Check sheet for the modelled part. Datum: model origin and axes. Units: mm. Face numbers are marked on the shaded views. A direction names the side the tool comes from. Coordinates: 2 decimals unless noted, no trailing zeros. Order: outer loops, then holes, each group sorted by start corner. A loop starts at its lowest first (then second) coordinate and runs counter-clockwise, first axis right, second up.
1. Draft check along Z on the marked faces 1, 2, 3 and 4. Enter one of: released by +Z, released by -Z, zero draft, split by the parting line, or undercut.
2. Cross-section at C-C (y = -49). Enter the section's corners in (x, z).
3. Gauge pin test, flat ends, axial feed: pin 1 Ø6 at (y, z) = (-22, 7) entering from +X; pin 2 Ø4 at (x, y) = (-5.5, -38) entering from -Z; pin 3 Ø1.5 at (y, z) = (-6.5, -3) entering from +X. Record the tip position at first contact, or that the pin passes through.
4. Set-up check for the marked faces 5 and 6: record each of +Z, -Z, +X, -X, +Y, -Y from which the full face is reachable in a straight line by a thin tool's end or side.
5. Cross-section at A-A (z = 0). Enter the section's corners in (x, y).
6. Cross-section at D-D (x = 6.75). Enter the section's corners in (y, z).
7. Cross-section at B-B (x = 0). Enter the section's corners in (y, z), then the cut area to 3 significant figures.
8. Thickness scan on line 1 (Z direction, x = 0, y = -0.1); line 2 (Z direction, x = 0, y = -17); line 3 (Y direction, x = 9.75, z = -3.5). Record the ranges inside material, lowest first.
```python
from build123d import *

# Parameters (mm, degrees)
F0_R     = 12
F1_DEPTH = 57.5
F2_R     = 7.5
F3_DEPTH = 2
F4_R     = 7.5
F5_DEPTH = 54
F6_R     = 4.25
F7_DEPTH = 8


with BuildPart() as f1:
    # F0 (on Front) → F1 (new body)
    with BuildSketch(Plane.XZ):
        Circle(F0_R)
    extrude(amount=F1_DEPTH)

    # F2 (on face) → F3 (join)
    with BuildSketch(Plane(origin=(0, 0, 0), x_dir=(-1, 0, 0), z_dir=(0, 1, 0))):
        Circle(F2_R)
    extrude(amount=F3_DEPTH)

    # F4 (on face) → F5 (cut)
    with BuildSketch(Plane.XZ.offset(57.5)):
        Circle(F4_R)
    extrude(amount=-F5_DEPTH, mode=Mode.SUBTRACT)

    # F6 (on face) → F7 (cut)
    with BuildSketch(Plane(origin=(0, 2, 0), x_dir=(-1, 0, 0), z_dir=(0, 1, 0))):
        Circle(F6_R)
    extrude(amount=-F7_DEPTH, mode=Mode.SUBTRACT)


solid = f1.part
```
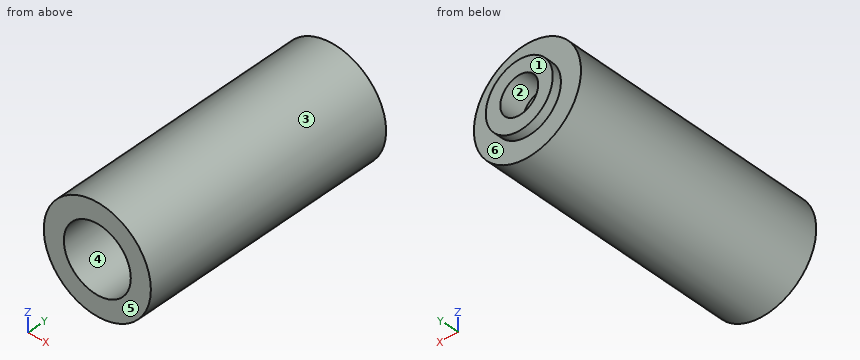
Data:
1. face 1: zero draft
1. face 2: undercut
1. face 3: split by the parting line
1. face 4: undercut
2. outline: circle Ø24 at (0, 0); hole circle Ø15 at (0, 0)
3. pin 1: stops at x = 11.31
3. pin 2: stops at z = -11.48
3. pin 3: stops at x = 11.79
4. face 5: +Z, -Z, +X, -X, -Y
4. face 6: +Y
5. outline: (-12, -57.5) - (-7.5, -57.5) - (-7.5, -3.5) - (-4.25, -3.5) - (-4.25, 2) - (-7.5, 2) - (-7.5, 0) - (-12, 0) - close; (4.25, -3.5) - (7.5, -3.5) - (7.5, -57.5) - (12, -57.5) - (12, 0) - (7.5, 0) - (7.5, 2) - (4.25, 2) - close
6. outline: (-57.5, -9.92) - (0, -9.92) - (0, -3.27) - (2, -3.27) - (2, 3.27) - (0, 3.27) - (0, 9.92) - (-57.5, 9.92) - (-57.5, 3.27) - (-3.5, 3.27) - (-3.5, -3.27) - (-57.5, -3.27) - close
7. outline: (-57.5, -12) - (0, -12) - (0, -7.5) - (2, -7.5) - (2, -4.25) - (-3.5, -4.25) - (-3.5, -7.5) - (-57.5, -7.5) - close; (-57.5, 7.5) - (-3.5, 7.5) - (-3.5, 4.25) - (2, 4.25) - (2, 7.5) - (0, 7.5) - (0, 12) - (-57.5, 12) - close
7. area: 553 mm2
8. line 1: z = -12 to -4.25, 4.25 to 12
8. line 2: z = -12 to -7.5, 7.5 to 12
8. line 3: y = -57.5 to 0
